Check sheet for the drawn part. Datum: minimum x, y, z corner. Units: mm. Round coordinates to 2 decimals unless told otherwise and drop trailing zeros. Write each loop counter-clockwise with the first axis right and the second up, starting at its lowest first coordinate (ties: lowest second). Pieces come first, ordered by that corner, then holes. Notation, with made-up numbers: (52.5, 9) - (71.5, 9) arc R27 ccw to (71.5, 46) - close; hole circle Ø9 at (-30.75, -15). An arc over 180 degrees is marked (long way). Answer as a JSON object with one key per item and string values. Group by question number.
1) Section check D-D (x = 4.5). Enter the section's corners in (y, z), then the cut area to 3 significant figures.
2) Section check C-C (y = 0.5). Enter the section's corners in (x, z), then the cut area to 3 significant figures.
3) Thickness scan on line 1 (Y direction, x = 3.75, z = 3.3); line 2 (X direction, y = 0.5, z = 2.6); line 3 (X direction, y = 3, z = 1.15). Record the ranges inside material, lowest first.
4) Go/stop test with a flat-tipped pin: pin 1 Ø1.5 at (x, y) = (4.5, 4) entering from +Z. Record where the tip stops, or that it passes through.
5) Mould release check, pull along Y, two halves, no side actions. Record for the marked faces 1, 2 and 3: +Y half, -Y half, draft (parallel to the pull), parting line (faces both ways), or undercut.
6) Section check B-B (z = 3.1). Enter the section's corners in (x, y).
7) Section check A-A (x = 3.75). Enter the section's corners in (y, z), then the cut area to 3 significant figures.
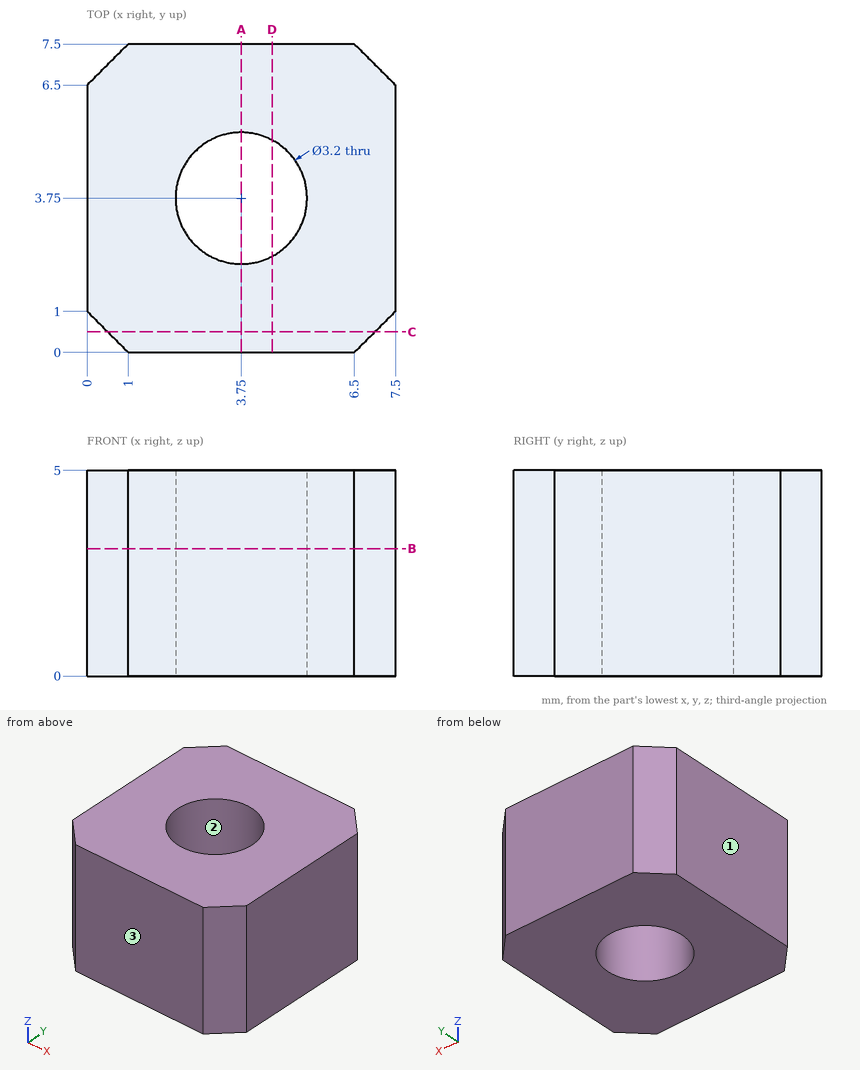
Returned:
{
 "1": {"outline": "(0, 0) - (2.34, 0) - (2.34, 5) - (0, 5) - close; (5.16, 0) - (7.5, 0) - (7.5, 5) - (5.16, 5) - close", "area": "23.4 mm2"},
 "2": {"outline": "(0.5, 0) - (7, 0) - (7, 5) - (0.5, 5) - close", "area": "32.5 mm2"},
 "3": {"line 1": "0 to 2.15, 5.35 to 7.5", "line 2": "0.5 to 7", "line 3": "0 to 2.34, 5.16 to 7.5"},
 "4": {"pin 1": "through"},
 "5": {"face 1": "draft", "face 2": "undercut", "face 3": "-Y half"},
 "6": {"outline": "(0, 1) - (1, 0) - (6.5, 0) - (7.5, 1) - (7.5, 6.5) - (6.5, 7.5) - (1, 7.5) - (0, 6.5) - close; hole circle Ø3.2 at (3.75, 3.75)"},
 "7": {"outline": "(0, 0) - (2.15, 0) - (2.15, 5) - (0, 5) - close; (5.35, 0) - (7.5, 0) - (7.5, 5) - (5.35, 5) - close", "area": "21.5 mm2"}
}
